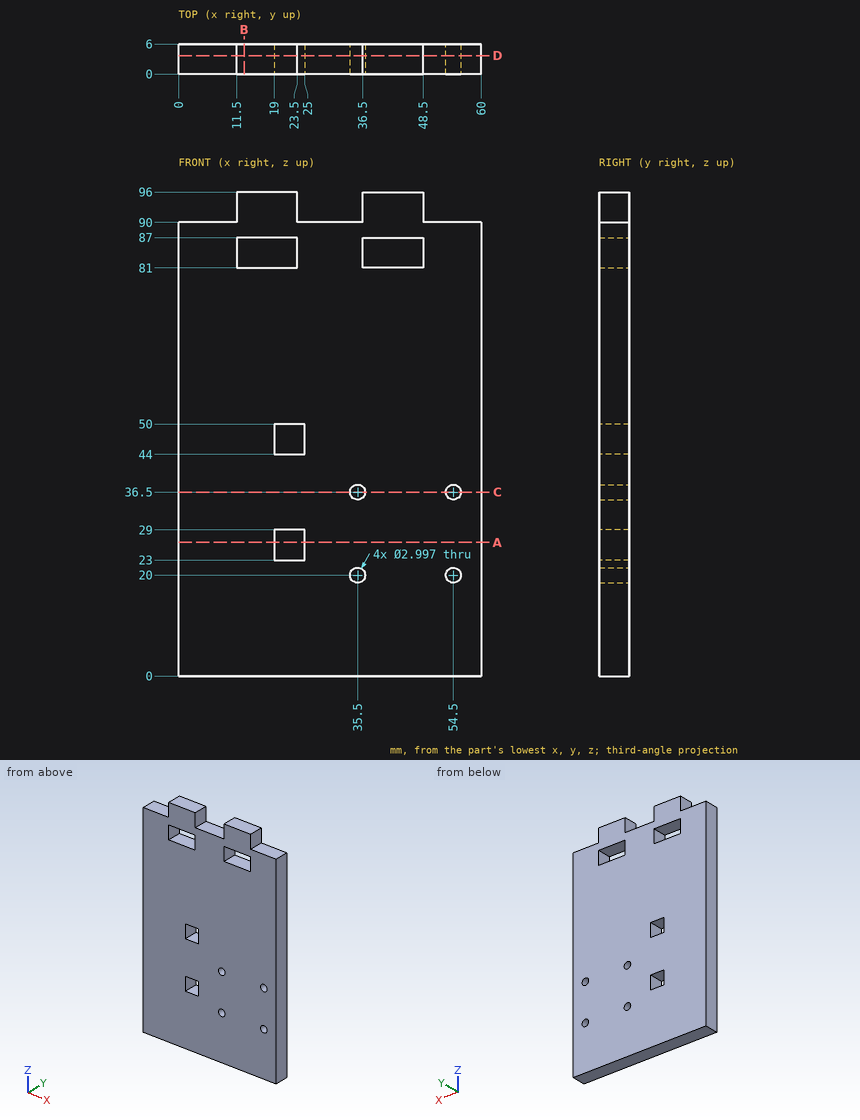
Answer from the drawing. Dimensions are ordinates in mm from the lowest x, y and z of the part. Coordinates: 2 decimals unless noted, no trailing zeros. Order: outer loops, then holes, each group sorted by start corner. A loop starts at its lowest first (then second) coordinate and runs counter-clockwise, first axis right, second up. Notation, with made-up numbers: (-18, -13) - (15, -13) arc R14 ccw to (15, -1) - close; hole circle Ø8 at (-36.75, 57). An arc over 180 degrees is marked (long way). Answer as a JSON object with one key per item and string values. Group by question number.
Item 1: Section C-C (z = 36.5) is taken. Give the vertices of the cut face in (x, y).
Item 2: Consider probe 1 along Z at (x, y) = (35.5, 2.9); probe 2 along X at (y, z) = (1.05, 83); probe 3 along X at (y, z) = (1.55, 20). Determine where each line is inside the solid, lowest interval first. Write a range as from..to.
Item 3: Flat-ended cylindrical pins translate along their axes: P1, Ø5, axis at x = 54.5, z = 20, coming from the +Y side; P2, Ø2.5, axis at x = 35.5, z = 36.5, coming from the -Y side. Find the tip coordinate at first contact, or state that the pin passes through.
Item 4: Section A-A (z = 26.5) is taken. Give the vertices of the cut face in (x, y), plus the area to 3 significant figures.
Item 5: Section D-D (y = 3.7) is taken. State how many separate pieces and enclosed holes the cut face has, plus the area to 3 significant figures.
Item 6: Section B-B (x = 13) is taken. Give the vertices of the cut face in (y, z).
Results are:
{
 "1": {"outline": "(0, 0) - (34, 0) - (34, 6) - (0, 6) - close; (37, 0) - (53, 0) - (53, 6) - (37, 6) - close; (56, 0) - (60, 0) - (60, 6) - (56, 6) - close"},
 "2": {"probe 1": "z = 0..18.5, 21.5..35, 38..90", "probe 2": "x = 0..11.5, 23.5..36.5, 48.5..60", "probe 3": "x = 0..34, 37..53, 56..60"},
 "3": {"P1": "stops at y = 6", "P2": "passes through"},
 "4": {"outline": "(0, 0) - (19, 0) - (19, 6) - (0, 6) - close; (25, 0) - (60, 0) - (60, 6) - (25, 6) - close", "area": "324 mm^2"},
 "5": {"separate pieces": "1", "enclosed holes": "8", "area": "5,300 mm^2"},
 "6": {"outline": "(0, 0) - (6, 0) - (6, 81) - (0, 81) - close; (0, 87) - (6, 87) - (6, 96) - (0, 96) - close"}
}
